Autodesk Inventor part; units mm, degrees
ref_plane "YZ Plane" through (0, 0, 0) normal (1, 0, 0) x (0, 1, 0)
ref_plane "XZ Plane" through (0, 0, 0) normal (0, 1, 0) x (-1, 0, 0)
ref_plane "XY Plane" through (0, 0, 0) normal (0, 0, 1) x (1, 0, 0)
sketch "Sketch1" plane through (0, 0, 0) normal (0, 0, 1) x (1, 0, 0)
  line L0 (-53.9497, 0) -> (53.9497, 0)
  line L1 (0, -8.2071) -> (0, 49.2426)
  line L2 (-37.5, 0) -> (37.5, 0)
  line L3 (37.5, 0) -> (37.5, 35)
  line L4 (32.5, 40) -> (-32.5, 40)
  line L5 (-37.5, 35) -> (-37.5, 0)
  arc A0 (-32.5, 40) -> (-37.5, 35) centre (-32.5, 35) ccw
  arc A1 (37.5, 35) -> (32.5, 40) centre (32.5, 35) ccw
  point P0 (0, 0)
  point P1 (37.5, 40)
  point P2 (-37.5, 40)
  dimension "d0" = 75
  dimension "d1" = 40
  dimension "d2" = 37.5
  dimension "d5" = 5
extrude "Extrusion1" add sketch "Sketch1" along normal blind 2.8
sketch "Sketch2" plane through (0, 0, 2.8) normal (0, 0, 1) x (1, 0, 0)
  line L0 (37.5, 0) -> (-37.5, 0)
  line L1 (37.5, 35) -> (37.5, 0)
  line L2 (-20, 0) -> (20, 0)
  line L3 (20, 0) -> (20, 5)
  line L4 (20, 5) -> (-20, 5)
  line L5 (-20, 5) -> (-20, 0)
  line L6 (-15.15, 22.4) -> (-15.15, 29.8)
  line L7 (-15.15, 29.8) -> (25.15, 29.8)
  line L8 (-21.15, 22.4) -> (-15.15, 22.4)
  line L9 (-21.15, 17.4) -> (-21.15, 22.4)
  line L10 (-15.15, 17.4) -> (-21.15, 17.4)
  line L11 (-15.15, 10) -> (-15.15, 17.4)
  line L12 (25.15, 10) -> (-15.15, 10)
  line L13 (25.15, 29.8) -> (25.15, 10)
  line L14 (-15.15, 29.8) -> (25.15, 29.8)
  point P0 (0, 0)
  dimension "d6" = 17.5
  dimension "d7" = 40
extrude "Extrusion2" cut sketch "Sketch2" against normal blind 10
sketch "Sketch3" plane through (0, 0, 2.8) normal (0, 0, 1) x (1, 0, 0)
  circle A0 centre (-19.5, 24.9) radius 2.5
  circle A1 centre (-19.5, 14.9) radius 2.5
  circle A2 centre (29.5, 14.9) radius 2.5
  circle A3 centre (29.5, 24.9) radius 2.5
  circle A4 centre (29.5, 14.9) radius 1.5
  circle A5 centre (29.5, 24.9) radius 1.5
  circle A6 centre (-19.5, 14.9) radius 1.5
  circle A7 centre (-19.5, 24.9) radius 1.5
  line L0 (-15.15, 17.4) -> (-21.15, 17.4)
  line L1 (29.3, 5.4) -> (29.3, 7)
  line L2 (32.5, 7) -> (32.5, 3.8)
  line L3 (29.3, 3.8) -> (29.3, 5.4)
  arc A8 (29.3, 3.8) -> (32.5, 3.8) centre (30.9, 3.8) ccw
  arc A9 (32.5, 7) -> (29.3, 7) centre (30.9, 7) ccw
  line L4 (-15.15, 10) -> (-15.15, 17.4)
  line L5 (-32.5, 5.4) -> (-32.5, 7)
  line L6 (-29.3, 7) -> (-29.3, 3.8)
  line L7 (-32.5, 3.8) -> (-32.5, 5.4)
  arc A10 (-29.3, 7) -> (-32.5, 7) centre (-30.9, 7) ccw
  arc A11 (-32.5, 3.8) -> (-29.3, 3.8) centre (-30.9, 3.8) ccw
  point P0 (0, 0)
  dimension "d10" = 3
  dimension "d11" = 3
  dimension "d12" = 3
  dimension "d13" = 3
extrude "Extrusion3" cut sketch "Sketch3" against normal through all contours A4 | A5 | A6 | A7 | L1 A9 L2 A8 L3 | L5 A10 L6 A11 L7
equation "\"d2\" = 0.5 * d0"
properties part number "Acrylic_YawServoSupport_1"
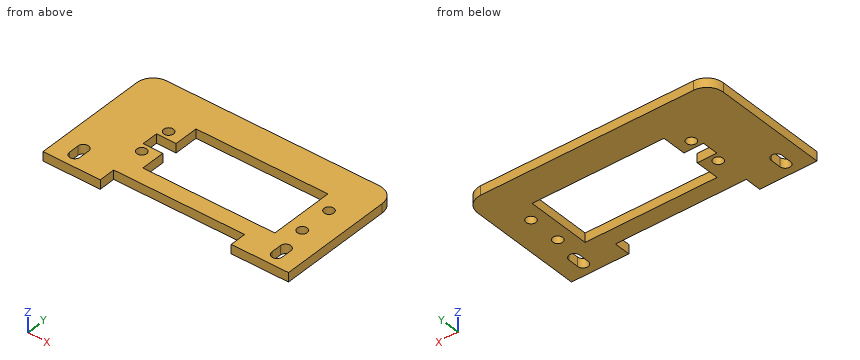
Work out the finished part from the listing and answer in its coordinate system (mm). Coordinates: 2 decimals unless noted, no trailing zeros. Write each loop counter-clockwise with the first axis right and the second up, starting at its lowest first coordinate (ties: lowest second). Pieces come first, ordered by that corner, then holes. Notation, with made-up numbers: (-19.75, 10) - (-15.75, 10) arc R24 cw to (-15.75, 31) - close; hole circle Ø7 at (-17, 1). An arc over 180 degrees is marked (long way). One line per question, with ' | ' between items.
1) Find section C-C, the plane z = 1. Give the number of separate pieces and of enclosed holes in the cut face, and give its area (3 significant figures).
Checks:
separate pieces: 1 | enclosed holes: 7 | area: 1,900 mm2
2) Find section B-B, the plane y = 11. Determine the outline of the cut face in (x, z), and give its area (3 significant figures).
Checks:
outline: (-37.5, 0) - (-15.15, 0) - (-15.15, 2.8) - (-37.5, 2.8) - close; (25.15, 0) - (37.5, 0) - (37.5, 2.8) - (25.15, 2.8) - close | area: 97.2 mm2
3) A flat-ended cylindrical pin translates along its axis: P1, Ø1.5, axis at x = 4.5, z = 2.5, coming from the -Y side. Find the tip coordinate at first contact, or state that the pin passes through.
Checks:
P1: y = 5
4) Consider probe 1 along Y at (x, z) = (-19.5, 2); probe 2 along Y at (x, z) = (29.5, 1.7); probe 3 along X at (y, z) = (14, 2.2). Determine where each line is inside the solid, lowest interval first. Write a range as [from, to].
Checks:
probe 1: [5, 13.4], [16.4, 17.4], [22.4, 23.4], [26.4, 40] | probe 2: [0, 3.03], [7.77, 13.4], [16.4, 23.4], [26.4, 40] | probe 3: [-37.5, -20.7], [-18.3, -15.15], [25.15, 28.3], [30.7, 37.5]
5) Find section A-A, the plane x = -30.9. Determine the outline of the cut face in (y, z), and give its area (3 significant figures).
Checks:
outline: (0, 0) - (2.2, 0) - (2.2, 2.8) - (0, 2.8) - close; (8.6, 0) - (40, 0) - (40, 2.8) - (8.6, 2.8) - close | area: 94.1 mm2
